from build123d import *

# Parameters (mm, degrees)
SKETCH1_R               = 2.55
BOSS_EXTRUDE1_DEPTH     = 18
SKETCH2_R               = 12.5
CUT_EXTRUDE1_DEPTH      = 3
SKETCH3_R               = 12.5
CUT_EXTRUDE2_DEPTH      = 3
SKETCH4_R               = 2.5
SKETCH4_R_2             = 1.6
CUT_EXTRUDE3_DEPTH      = 16
SKETCH5_W               = 11
SKETCH5_H               = 40
CUT_EXTRUDE4_DEPTH      = 21
CUT_EXTRUDE4_DEPTH_BACK = 21
SKETCH7_W               = 40
SKETCH7_H               = 58
CUT_EXTRUDE5_DEPTH      = 10
SKETCH8_R               = 2.1
SKETCH8_W               = 25
SKETCH8_H               = 42
CUT_EXTRUDE6_DEPTH      = 9


with BuildPart() as part:
    # Sketch1 → Boss-Extrude1 (new body)
    with BuildSketch(Plane.XY):
        with BuildLine():
            ThreePointArc((20, 110), (0, 130), (-20, 110))
            Line((-20, 110), (-15, 0))
            ThreePointArc((-15, 0), (0, -15), (15, 0))
            Line((15, 0), (20, 110))
        make_face()
        Circle(SKETCH1_R, mode=Mode.SUBTRACT)
    extrude(amount=BOSS_EXTRUDE1_DEPTH)

    # Sketch2 → Cut-Extrude1 (cut)
    with BuildSketch(Plane.XY.offset(18)):
        with Locations((0, 110)):
            Circle(SKETCH2_R)
    extrude(amount=-CUT_EXTRUDE1_DEPTH, mode=Mode.SUBTRACT)

    # Sketch3 → Cut-Extrude2 (cut)
    with BuildSketch(Plane(origin=(0, 0, 0), x_dir=(-1, 0, 0), z_dir=(0, 0, -1))):
        with Locations((0, 110)):
            Circle(SKETCH3_R)
    extrude(amount=-CUT_EXTRUDE2_DEPTH, mode=Mode.SUBTRACT)

    # Sketch4 → Cut-Extrude3 (cut, through all)
    with BuildSketch(Plane.XY.offset(15)):
        with Locations((0, 110)):
            Circle(SKETCH4_R)
        with Locations((-5, 115)):
            Circle(SKETCH4_R_2)
        with Locations((-5, 105)):
            Circle(SKETCH4_R_2)
        with Locations((5, 105)):
            Circle(SKETCH4_R_2)
        with Locations((5, 115)):
            Circle(SKETCH4_R_2)
    extrude(amount=-CUT_EXTRUDE3_DEPTH, mode=Mode.SUBTRACT)

    # Sketch5 → Cut-Extrude4 (cut, two sides)
    with BuildSketch(Plane(origin=(0, 0, 0), x_dir=(0, 0, -1), z_dir=(1, 0, 0))) as cut_extrude4_sk:
        with Locations((-9, 5)):
            Rectangle(SKETCH5_W, SKETCH5_H)
    extrude(amount=CUT_EXTRUDE4_DEPTH, mode=Mode.SUBTRACT)
    extrude(cut_extrude4_sk.sketch, amount=-CUT_EXTRUDE4_DEPTH_BACK, mode=Mode.SUBTRACT)

    # Sketch7 → Cut-Extrude5 (cut)
    with BuildSketch(Plane.XY.offset(18)):
        with Locations((0, 61)):
            Rectangle(SKETCH7_W, SKETCH7_H)
    extrude(amount=-CUT_EXTRUDE5_DEPTH, mode=Mode.SUBTRACT)

    # Sketch8 → Cut-Extrude6 (cut, through all)
    with BuildSketch(Plane.XY.offset(8)):
        with Locations((-5, 85)):
            Circle(SKETCH8_R)
        with Locations((5, 85)):
            Circle(SKETCH8_R)
        with Locations((5, 37)):
            Circle(SKETCH8_R)
        with Locations((-5, 37)):
            Circle(SKETCH8_R)
        with Locations((0, 61)):
            Rectangle(SKETCH8_W, SKETCH8_H)
    extrude(amount=-CUT_EXTRUDE6_DEPTH, mode=Mode.SUBTRACT)


solid = part.part
Source: CAD feature listing. Evaluate the final solid. Frame: model axes, mm. A direction names the side the tool comes from. Coordinates: 2 decimals unless noted, no trailing zeros. Loops run counter-clockwise (first coordinate to the right, second up) from the corner with the lowest first, then second, coordinate; pieces in that order, holes last. Notation, with made-up numbers: (58, 70) - (88, 70) arc R22 ccw to (88, 87) - close; hole circle Ø10 at (46.5, -38). An arc over 180 degrees is marked (long way). Return JSON: item names as keys, results as strings.
Q1. Section B-B, the plane y = 22. Return loops of the section in (x, z), plus the area to 3 significant figures.
Results:
{"outline": "(-16, 0) - (16, 0) - (16, 3.5) - (-16, 3.5) - close; (-16, 14.5) - (16, 14.5) - (16, 18) - (-16, 18) - close", "area": "224 mm2"}
Q2. Section A-A, the plane z = 9.5. Return loops of the section in (x, y).
Results:
{"outline": "(-20, 110) - (-19.09, 90) - (19.09, 90) - (20, 110) arc R20 ccw to start; (-16.45, 32) - (-16.14, 25) - (16.14, 25) - (16.45, 32) - close; hole circle Ø3.2 at (-5, 105); hole circle Ø3.2 at (-5, 115); hole circle Ø5 at (0, 110); hole circle Ø3.2 at (5, 105); hole circle Ø3.2 at (5, 115)"}
Q3. Section D-D, the plane x = 5. Give the number of separate pieces and of enclosed holes in the cut face, plus the area to 3 significant figures.
Results:
{"separate pieces": "6", "enclosed holes": "0", "area": "955 mm2"}
Q4. Section C-C, the plane y = 105. Return loops of the section in (x, z).
Results:
{"outline": "(-19.77, 0) - (-11.46, 0) - (-11.46, 3) - (-6.6, 3) - (-6.6, 15) - (-11.46, 15) - (-11.46, 18) - (-19.77, 18) - close; (-3.4, 3) - (3.4, 3) - (3.4, 15) - (-3.4, 15) - close; (6.6, 3) - (11.46, 3) - (11.46, 0) - (19.77, 0) - (19.77, 18) - (11.46, 18) - (11.46, 15) - (6.6, 15) - close"}
Q5. Contact query for flat-ended pins moving along their axis: P1, Ø6, axis at y = 25, z = 15, coming from the -X side; P2, Ø10, axis at x = -3.5, z = 7, coming from the -Y side; P3, Ø15, axis at x = 0, y = 110, coming from the +Z side; P4, Ø5, axis at x = 2, z = 10.5, coming from the +Y side. Output: stop coordinate, or through.
Results:
{"P1": "x = -16.27", "P2": "y = -15", "P3": "z = 15", "P4": "y = 130"}
Q6. Material intervals for line 1 along Y through (x, z) = (0, 1.4); line 2 along Y through (x, z) = (0, 17.1); line 3 along Y through (x, z) = (10.5, 17), sorted ascending.
Results:
{"line 1": "-15 to -2.55, 2.55 to 40, 82 to 97.5, 122.5 to 130", "line 2": "-15 to -2.55, 2.55 to 32, 90 to 97.5, 122.5 to 130", "line 3": "-10.71 to 32, 90 to 103.22, 116.78 to 127.02"}
Q7. Access query for faces 4 (the cylindrical face through (1.627, 122.394, 1.479)), 5 (the flat face through (-13, 68, 8)), 6 (the flat face through (0, 82, 4)), 7 (the flat face through (0, 5, 14.5)). Directions: +Z, -Z, +X, -X, +Y, -Y. A direction counts if a zero-diameter tool reaches every point of the face in a straight line with its end or side. Return the directions, or none.
Results:
{"face 4": "-Z", "face 5": "+Z, +X, -X", "face 6": "+Z, -Z", "face 7": "+X, -X, -Y"}
Q8. Mould query, pull axis X, two halves, no side actions, for faces 1 (the flat face through (-17.535, 55.77, 6.874)), 2 (the flat face through (0, 25, 9)), 3 (the cylindrical face through (4.792, 116.586, 9.084)). Classes: released by +X, released by -X, zero draft, split by the parting line, or undercut.
Results:
{"face 1": "released by -X", "face 2": "zero draft", "face 3": "undercut"}
